The model under review builds one solid part; all positions refer to its coordinate system, in mm. Coordinates: 2 decimals unless noted, no trailing zeros. Order: outer loops, then holes, each group sorted by start corner. A loop starts at its lowest first (then second) coordinate and runs counter-clockwise, first axis right, second up. Notation, with made-up numbers: M -1,19.25 L 6,19.25 A23 cw 6,52.25 Z; hole C 32,64.25 d3. An arc over 180 degrees is marked long. Write each question's results on one line, items separated by ' | '.
Autodesk Inventor part; units mm, degrees
ref_plane "YZ Plane" through (0, 0, 0) normal (1, 0, 0) x (0, 1, 0)
ref_plane "XZ Plane" through (0, 0, 0) normal (0, 1, 0) x (-1, 0, 0)
ref_plane "XY Plane" through (0, 0, 0) normal (0, 0, 1) x (1, 0, 0)
sketch "Sketch1" plane through (0, 0, 0) normal (0, 1, 0) x (-1, 0, 0)
  circle A0 centre (59.9806, -102.3601) radius 22.5
  circle A1 centre (61.712, -54.745) radius 19.25
  circle A2 centre (65.7506, -15.2725) radius 16
  circle A3 centre (22.7676, -23.4976) radius 22.5
  circle A4 centre (20.1892, -68.6854) radius 19.25
  circle A5 centre (17.0449, -106.5008) radius 16
  line L0 (-7.557, 11.8403) -> (92.5214, 11.8403)
  line L1 (92.5214, 11.8403) -> (92.5214, -134.0855)
  line L2 (92.5214, -134.0855) -> (-7.557, -134.0855)
  line L3 (-7.557, -134.0855) -> (-7.557, 11.8403)
  point P0 (0, 0)
extrude "Extrusion1" add sketch "Sketch1" along normal blind 3
properties part number "Center"
1) Take a section at B-B on x = -55.5. State the section outline as (y, z) points.
Solutions:
outline: M 0,-134.09 L 3,-134.09 L 3,-124.41 L 0,-124.41 Z; M 0,-80.31 L 3,-80.31 L 3,-72.97 L 0,-72.97 Z; M 0,-36.52 L 3,-36.52 L 3,-27.56 L 0,-27.56 Z; M 0,-2.99 L 3,-2.99 L 3,11.84 L 0,11.84 Z
2) For pin 1 (10 mm diameter, centred on x = -8.5, z = -26, fed in from -Y), flat-tipped, find the tip position at first contact; note if it passes through.
Solutions:
pin 1: through
3) To check wall thickness, follow line 1 along X through (y, z) = (1.75, -60); line 2 along X through (y, z) = (2.8, -110); line 3 along Z through (x, y) = (-20.5, 2.85). State the ranges of each line that lie inside material, in increasing order.
Solutions:
line 1: -92.52 to -80.23, -43.19 to -37.37, -3.01 to 7.56 | line 2: -92.52 to -81.14, -38.82 to -32.66, -1.43 to 7.56 | line 3: -134.09 to -122.12, -90.88 to -87.93, -49.44 to -45.88, -1.11 to 11.84
4) The part is to be moulded in two halves that separate along X. For faces 1 (the cylindrical face through (-53.05, 1.48, -5.54)), 2 (the flat face through (7.557, 1, -62)), 3 (the flat face through (-42, 1, 11.84)), 4 (the cylindrical face through (-29.072, 1.479, -51.607)), say which applies: pulls with the +X half, pulls with the -X half, needs draft (parallel to the pull), parting line crosses it, or undercut.
Solutions:
face 1: undercut | face 2: pulls with the +X half | face 3: needs draft | face 4: undercut
5) Take a section at D-D on y = 1.2. Count the separate pieces of the cut face and the enclosed holes in it, plus the area to 3 significant figures.
Solutions:
separate pieces: 1 | enclosed holes: 6 | area: 7,490 mm2
6) Take a section at A-A on z = -11. State the section outline as (x, y) points.
Solutions:
outline: M -92.52,0 L -81.17,0 L -81.17,3 L -92.52,3 Z; M -50.33,0 L -41.48,0 L -41.48,3 L -50.33,3 Z; M -4.06,0 L 7.56,0 L 7.56,3 L -4.06,3 Z
7) Take a section at C-C on z = -33.5. State the section outline as (x, y) points, plus the area to 3 significant figures.
Solutions:
outline: M -92.52,0 L -42.92,0 L -42.92,3 L -92.52,3 Z; M -2.61,0 L 7.56,0 L 7.56,3 L -2.61,3 Z | area: 179 mm2
